Verification items for the finished model (mm, model axes). A direction names the side the tool comes from. Round coordinates to 2 decimals unless told otherwise and drop trailing zeros. Write each loop counter-clockwise with the first axis right and the second up, starting at its lowest first coordinate (ties: lowest second). Pieces come first, ordered by that corner, then holes. Notation, with made-up numbers: (-17, 41) - (41, 41) arc R23 ccw to (41, 50) - close; hole circle Ø5 at (33.5, 79). An arc over 180 degrees is marked (long way). Answer as a JSON object with one key per item and string values. Group by question number.
1) Section check C-C (x = 0). Enter the section's corners in (y, z).
2) Section check D-D (x = -135). Enter the section's corners in (y, z), then the cut area to 3 significant figures.
3) Section check A-A (z = 13). Enter the section's corners in (x, y), then the cut area to 3 significant figures.
4) Thickness scan on line 1 (Y direction, x = -80, z = 3); line 2 (Y direction, x = -0.5, z = 29); line 3 (Z direction, x = -5, y = 66). Record the ranges inside material, lowest first.
5) Section check B-B (y = 0). Enter the section's corners in (x, z).
6) Go/stop test with flat-tipped pins: pin 1 Ø24 at (x, y) = (-2.5, 89) entering from -Z; pin 2 Ø15 at (x, y) = (-85.5, 0) entering from +Z; pin 3 Ø12 at (x, z) = (-26.5, 52) entering from -Y; pin 4 Ø8 at (y, z) = (-10.5, 8) entering from -X. Record where each tip stops, or that it passes through.
7) Set-up check for faces 1 (the flat face through (-98, -15.06, 3)), 2 (the flat face through (17.673, 98, 68)), 3 (the flat face through (-98, 14.94, 3)), 4 (the flat face through (-150, 0, 3)), 5 (the flat face through (-29, 1, 0)): record each of +Z, -Z, +X, -X, +Y, -Y from which the full face is reachable in a straight line by a thin tool's end or side.
```python
from build123d import *

# Parameters (mm, degrees)
SKETCH1_R           = 50
BOSS_EXTRUDE1_DEPTH = 70
SKETCH2_W           = 30
SKETCH2_H           = 5
BOSS_EXTRUDE2_DEPTH = 150
SKETCH4_W           = 5
SKETCH4_H           = 30
BOSS_EXTRUDE3_DEPTH = 150


with BuildPart() as part:
    # Sketch1 → Boss-Extrude1 (new body)
    with BuildSketch(Plane.XY):
        Circle(SKETCH1_R)
    extrude(amount=BOSS_EXTRUDE1_DEPTH)

    # Sketch2 → Boss-Extrude2 (add)
    with BuildSketch(Plane(origin=(0, 0, 0), x_dir=(1, 0, 0), z_dir=(0, 1, 0))):
        with Locations((2.673304283, -67.5)):
            Rectangle(SKETCH2_W, SKETCH2_H)
    extrude(amount=BOSS_EXTRUDE2_DEPTH)

    # Sketch4 → Boss-Extrude3 (add)
    with BuildSketch(Plane(origin=(0, 0, 0), x_dir=(0, 0, -1), z_dir=(1, 0, 0))):
        with Locations((-2.5, -0.059930336)):
            Rectangle(SKETCH4_W, SKETCH4_H)
    extrude(amount=-BOSS_EXTRUDE3_DEPTH)


solid = part.part
```
Returned:
{
 "1": {"outline": "(-50, 0) - (50, 0) - (50, 65) - (150, 65) - (150, 70) - (-50, 70) - close"},
 "2": {"outline": "(-15.06, 0) - (14.94, 0) - (14.94, 5) - (-15.06, 5) - close", "area": "150 mm2"},
 "3": {"outline": "circle Ø100 at (0, 0)", "area": "7,850 mm2"},
 "4": {"line 1": "-15.06 to 14.94", "line 2": "-50 to 50", "line 3": "65 to 70"},
 "5": {"outline": "(-150, 0) - (50, 0) - (50, 70) - (-50, 70) - (-50, 5) - (-150, 5) - close"},
 "6": {"pin 1": "z = 65", "pin 2": "z = 5", "pin 3": "y = -45.6", "pin 4": "x = -150"},
 "7": {"face 1": "+Z, -Z, -X, -Y", "face 2": "+Z, -Z, +X, +Y", "face 3": "+Z, -Z, -X, +Y", "face 4": "+Z, -Z, -X, +Y, -Y", "face 5": "-Z, +X, -X, +Y, -Y"}
}
